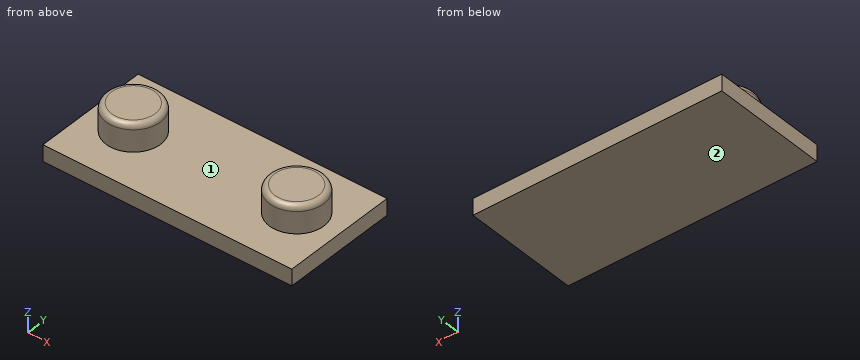
```python
from build123d import *

# Parameters (mm, degrees)
SKETCH1_W           = 45.7
SKETCH1_H           = 21.3
BOSS_EXTRUDE1_DEPTH = 3
SKETCH2_R           = 5
BOSS_EXTRUDE2_DEPTH = 5
FILLET1_R           = 1


with BuildPart() as part:
    # Sketch1 → Boss-Extrude1 (new body)
    with BuildSketch(Plane.XY):
        Rectangle(SKETCH1_W, SKETCH1_H)
    extrude(amount=BOSS_EXTRUDE1_DEPTH)

    # Sketch2 → Boss-Extrude2 (add)
    with BuildSketch(Plane.XY.offset(3)):
        with Locations(Location((-15, 0, 0), (0, 0, 180))):
            Circle(SKETCH2_R)
        with Locations(Location((15, 0, 0), (0, 0, 180))):
            Circle(SKETCH2_R)
    extrude(amount=BOSS_EXTRUDE2_DEPTH)

    # Fillet1
    fillet1_edges = [part.edges().sort_by_distance(p)[0] for p in [
        (-10, 0, 8),
        (20, 0, 8),
    ]]
    fillet(fillet1_edges, radius=FILLET1_R)


solid = part.part
```
Geometry: final body of the model. Coordinates: model frame, mm. Face numbers are marked on the shaded views. A direction names the side the tool comes from. Give positions to 0.01 mm unless a question says otherwise; leave off trailing zeros. Loops run counter-clockwise (first coordinate to the right, second up) from the corner with the lowest first, then second, coordinate; pieces in that order, holes last. Notation, with made-up numbers: (40.25, 50.5) -> (67.25, 50.5) arc R23 cw to (67.25, 77.5) -> close; hole circle Ø8 at (87.5, -37). An arc over 180 degrees is marked (long way). Use CSV: the item, a comma, the result in double quotes.
(1) Cut plane A-A (x = -15). Output: boundary loops of the cut face in (y, z), plus the area to 3 significant figures.
From the geometry:
outline,"(-10.65, 0) -> (10.65, 0) -> (10.65, 3) -> (5, 3) -> (5, 7) arc R1 ccw to (4, 8) -> (-4, 8) arc R1 ccw to (-5, 7) -> (-5, 3) -> (-10.65, 3) -> close"
area,"113 mm^2"
(2) Cut plane B-B (y = 0). Output: boundary loops of the cut face in (x, z), plus the area to 3 significant figures.
From the geometry:
outline,"(-22.85, 0) -> (22.85, 0) -> (22.85, 3) -> (20, 3) -> (20, 7) arc R1 ccw to (19, 8) -> (11, 8) arc R1 ccw to (10, 7) -> (10, 3) -> (-10, 3) -> (-10, 7) arc R1 ccw to (-11, 8) -> (-19, 8) arc R1 ccw to (-20, 7) -> (-20, 3) -> (-22.85, 3) -> close"
area,"236 mm^2"
(3) Cut plane D-D (x = -7.5). Output: boundary loops of the cut face in (y, z).
From the geometry:
outline,"(-10.65, 0) -> (10.65, 0) -> (10.65, 3) -> (-10.65, 3) -> close"
(4) Cut plane C-C (z = 3.5). Output: boundary loops of the cut face in (x, y), plus the area to 3 significant figures.
From the geometry:
outline,"circle Ø10 at (-15, 0); circle Ø10 at (15, 0)"
area,"157 mm^2"
(5) Access query for the marked faces 1 and 2. Directions: +Z, -Z, +X, -X, +Y, -Y. A direction counts if a zero-diameter tool reaches every point of the face in a straight line with its end or side. Return the directions, or none.
From the geometry:
face 1,"+Z"
face 2,"-Z, +X, -X, +Y, -Y"
(6) Ray query, line 1 along Y through (x, z) = (-12, 3.5); line 2 along Z through (x, y) = (4, 1.25); line 3 along X through (y, z) = (4, 3.5). Return the intervals inside material, ascending. Write a range as [from, to].
From the geometry:
line 1,"[-4, 4]"
line 2,"[0, 3]"
line 3,"[-18, -12], [12, 18]"
(7) First-contact query: P1, Ø6.5, axis at x = 7.5, y = -1, coming from the +Z side; P2, Ø2, axis at x = -3, y = 5, coming from the +Z side; P3, Ø1, axis at y = 4.5, z = 7, coming from the +X side. Flat tips, straight axial feed; report the tip coordinate or a pass-through.
From the geometry:
P1,"z = 7.95"
P2,"z = 3"
P3,"x = 18"
